Here's the drawing with two shaded views (mm, measured from the low corner). I have some questions. A direction names the side the tool comes from. Round coordinates to 2 decimals unless told otherwise and drop trailing zeros. Loops run counter-clockwise (first coordinate to the right, second up) from the corner with the lowest first, then second, coordinate; pieces in that order, holes last. Notation, with made-up numbers: (8, 45) - (43, 45) arc R11 cw to (43, 52) - close; hole circle Ø8 at (82, -8.75). An arc over 180 degrees is marked (long way). Use one line per item in the form item = value.
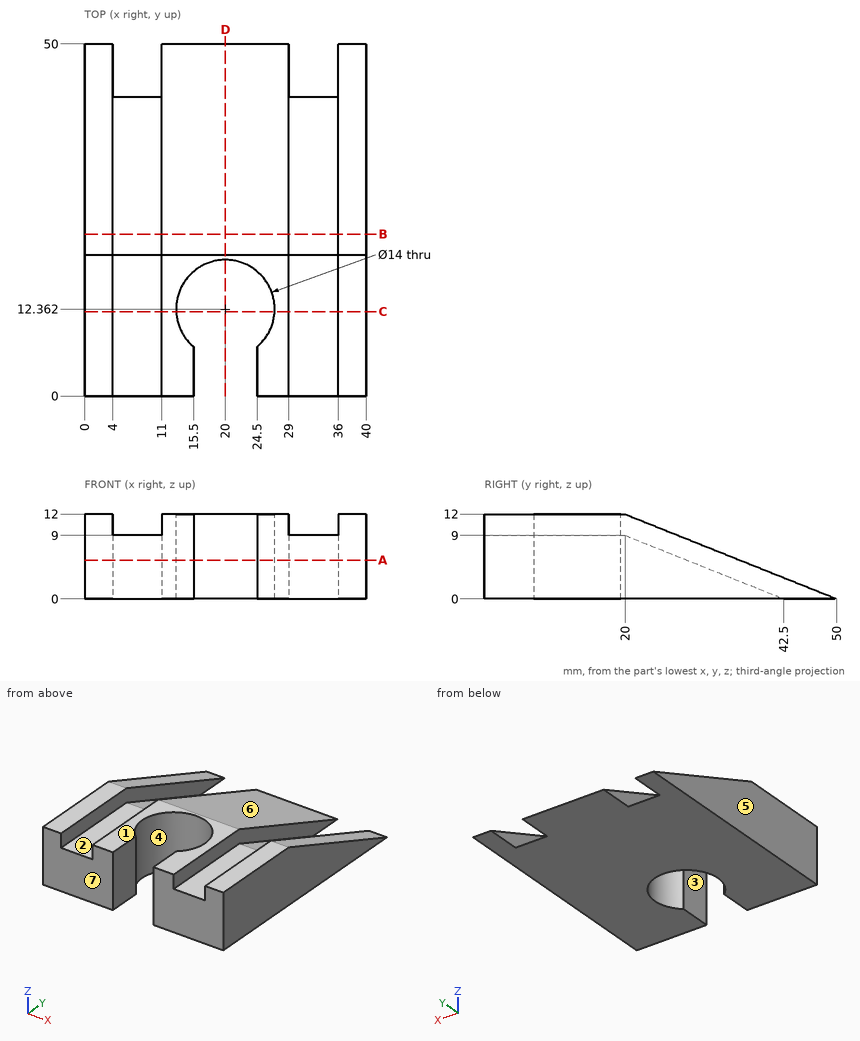
1. We'd pull the mould along Y, two halves only. Please class the marked faces 4, 5, 6 and 7: +Y half, -Y half, draft (parallel to the pull), parting line (faces both ways), or undercut.
Solution:
face_4 = undercut
face_5 = draft
face_6 = +Y half
face_7 = -Y half
2. If we section it at B-B, the plane y = 23: Write out the boundary of the cut face in (x, z).
Solution:
outline = (0, 0) - (40, 0) - (40, 10.8) - (36, 10.8) - (36, 7.8) - (29, 7.8) - (29, 10.8) - (11, 10.8) - (11, 7.8) - (4, 7.8) - (4, 10.8) - (0, 10.8) - close
3. For P1, Ø5.5, axis at x = 32.5, y = 8, coming from the +Z side; P2, Ø1.5, axis at y = 40.5, z = 6.5, coming from the +X side, each with a flat end and sliding along its axis, tell me the tip position at first contact or that it passes through.
Solution:
P1 = 9
P2 = through
4. If we section it at D-D, the plane x = 20: Write out the boundary of the cut face in (y, z), plus the area to 3 significant figures.
Solution:
outline = (19.36, 0) - (50, 0) - (20, 12) - (19.36, 12) - close
area = 188 mm^2
5. Please list where these lines run through material, in increasing order: line 1 along X through (y, z) = (36.5, 4); line 2 along X through (y, z) = (2, 6.5); line 3 along Z through (x, y) = (2, 27.5).
Solution:
line_1 = 0 to 4, 11 to 29, 36 to 40
line_2 = 0 to 15.5, 24.5 to 40
line_3 = 0 to 9
6. If we section it at C-C, the plane y = 12: Write out the boundary of the cut face in (x, z), plus the area to 3 significant figures.
Solution:
outline = (0, 0) - (13.01, 0) - (13.01, 12) - (11, 12) - (11, 9) - (4, 9) - (4, 12) - (0, 12) - close; (26.99, 0) - (40, 0) - (40, 12) - (36, 12) - (36, 9) - (29, 9) - (29, 12) - (26.99, 12) - close
area = 270 mm^2
7. On a 3-axis mill with a long thin cutter (end or side, diameter ignored), from which of +Z, -Z, +X, -X, +Y, -Y can I reach the whole of each face in a straight line? I mean the marked faces 1, 2 and 3. Say none if no direction works.
Solution:
face_1 = +Z, +X, -X, +Y, -Y
face_2 = +Z, +Y, -Y
face_3 = +Z, -Z, -Y
8. If we section it at A-A, the plane z = 5.5: Write out the boundary of the cut face in (x, y), plus the area to 3 significant figures.
Solution:
outline = (0, 0) - (15.5, 0) - (15.5, 7) arc R7 cw (long way) to (24.5, 7) - (24.5, 0) - (40, 0) - (40, 36.25) - (36, 36.25) - (36, 28.75) - (29, 28.75) - (29, 36.25) - (11, 36.25) - (11, 28.75) - (4, 28.75) - (4, 36.25) - (0, 36.25) - close
area = 1,140 mm^2
